Input: part model. Units: mm. Frame: model coordinates. A direction names the side the tool comes from. Round coordinates to 2 decimals unless told otherwise and drop trailing zeros. Loops run counter-clockwise (first coordinate to the right, second up) from the corner with the lowest first, then second, coordinate; pieces in that order, holes last. Notation, with made-up numbers: (79.5, -14) - (133.5, -14) arc R14 cw to (133.5, 6) - close; hole circle Ø9 at (-22.5, 58). An arc over 180 degrees is marked (long way). One line per question, with ' | ' between items. Start each with the question number.
from build123d import *

# Parameters (mm, degrees)
SKETCH2_W           = 141.2875
SKETCH2_H           = 157.1625
BOSS_EXTRUDE1_DEPTH = 12.7
SHELL1_T            = -6.35


with BuildPart() as part:
    # Sketch2 → Boss-Extrude1 (new body)
    with BuildSketch(Plane.XY):
        Rectangle(SKETCH2_W, SKETCH2_H)
    extrude(amount=BOSS_EXTRUDE1_DEPTH)

    # Shell1
    shell1_openings = [part.faces().sort_by_distance(p)[0] for p in [
        (0, 0, 12.7),
    ]]
    offset(amount=SHELL1_T, openings=shell1_openings, kind=Kind.INTERSECTION)


solid = part.part
(1) Pin query (flat end, axial travel): P1, Ø1, axis at x = 24.5, y = 42.5, coming from the -Z side; P2, Ø8, axis at x = 52.5, y = -56.5, coming from the +Z side. Return the tip coordinate at first contact, or that it passes through.
(2) Pull-direction query (X, two-part tool) for faces 3 (the face through (64.294, -1, 9)), 4 (the face through (70.644, -1, 6)), 5 (the face through (-70.644, -1, 6)); classes: released by +X, released by -X, zero draft, split by the parting line, or undercut.
(3) Line query: line 1 along X through (y, z) = (-52, 8); line 2 along Y through (x, z) = (-19.5, 12.25); line 3 along Z through (x, y) = (-49, 34.5). Output: solid intervals per line, ascending. Write a range as from..to.
(4) Section A-A, the plane z = 10.25. Output: boundary loops of the cut face in (x, y), plus the area to 3 significant figures.
(5) Reachability of faces 1 (the face through (-1, -72.231, 9)), 2 (the face through (-1, 1, 0)) from +Z, -Z, +X, -X, +Y, -Y: full face, straight path, thin tool, end or side. Return the list, or none.
(6) Section B-B, the plane y = -42.5. Output: boundary loops of the cut face in (x, z).
(7) Section C-C, the plane x = -7.5. Output: boundary loops of the cut face in (y, z), plus the area to 3 significant figures.
Derived:
1) P1: stops at z = 0 | P2: stops at z = 6.35
2) face 3: undercut | face 4: released by +X | face 5: released by -X
3) line 1: x = -70.64..-64.29, 64.29..70.64 | line 2: y = -78.58..-72.23, 72.23..78.58 | line 3: z = 0..6.35
4) outline: (-70.64, -78.58) - (70.64, -78.58) - (70.64, 78.58) - (-70.64, 78.58) - close; hole (-64.29, -72.23) - (64.29, -72.23) - (64.29, 72.23) - (-64.29, 72.23) - close | area: 3,630 mm²
5) face 1: +Z | face 2: -Z, +X, -X, +Y, -Y
6) outline: (-70.64, 0) - (70.64, 0) - (70.64, 12.7) - (64.29, 12.7) - (64.29, 6.35) - (-64.29, 6.35) - (-64.29, 12.7) - (-70.64, 12.7) - close
7) outline: (-78.58, 0) - (78.58, 0) - (78.58, 12.7) - (72.23, 12.7) - (72.23, 6.35) - (-72.23, 6.35) - (-72.23, 12.7) - (-78.58, 12.7) - close | area: 1,080 mm²
